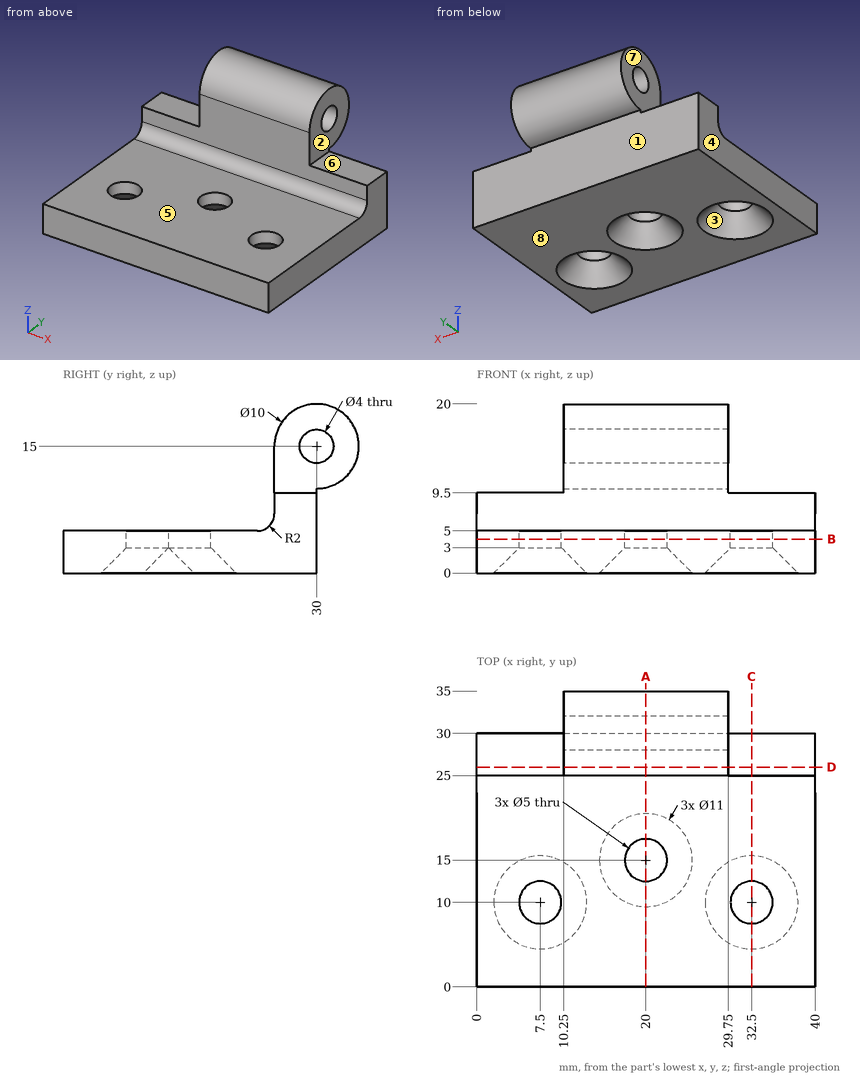
Study the drawing (mm; zero at the part's minimum x, y, z) and answer. A direction names the side the tool comes from. Round coordinates to 2 decimals unless told otherwise and drop trailing zeros. Loops run counter-clockwise (first coordinate to the right, second up) from the corner with the lowest first, then second, coordinate; pieces in that order, holes last.
Q1. Section C-C, the plane x = 32.5 is taken. Determine the outline of the cut face in (y, z), then the cut area to 3 significant figures.
Q2. Section D-D, the plane y = 26 is taken. Determine the outline of the cut face in (x, z), then the cut area to 3 significant figures.
Q3. Section B-B, the plane z = 4 is taken. Determine the outline of the cut face in (x, y), then the cut area to 3 significant figures.
Q4. Section A-A, the plane x = 20 is taken. Determine the outline of the cut face in (y, z).
Q5. For a pull along X with two mould halves and no side action, classify the marked faces 1, 2 and 3 as released by +X, released by -X, zero draft, split by the parting line, or undercut.
Q6. Given pin 1 Ø2.5 at (x, z) = (17, 11) entering from -Y; pin 2 Ø3 at (x, y) = (32.5, 10) entering from -Z; pin 3 Ø11 at (y, z) = (31, 15.5) entering from -X; pin 4 Ø4 at (x, y) = (4, 6.5) entering from +Z, each flat-ended and moving along its own axis, determine where each tip first touches the part or whether it passes through.
Q7. Which of the six approach directions +Z, -Z, +X, -X, +Y, -Y give full straight-line access (tool end or side, diameter ignored) to the marked faces 4, 5, 6, 7 and 8?
Q8. Find the intervals of material crossed by line 1 (X direction, y = 10, z = 3.4); line 2 (Y direction, x = 32.5, z = 4.55); line 3 (Y direction, x = 25.5, z = 15), in increasing order.
Completed:
1. outline: (0, 0) - (4.5, 0) - (7.5, 3) - (7.5, 5) - (0, 5) - close; (12.5, 3) - (15.5, 0) - (30, 0) - (30, 9.5) - (25, 9.5) - (25, 7) arc R2 cw to (23, 5) - (12.5, 5) - close
1. area: 139 mm2
2. outline: (0, 0) - (40, 0) - (40, 9.5) - (29.75, 9.5) - (29.75, 18) - (10.25, 18) - (10.25, 9.5) - (0, 9.5) - close
2. area: 546 mm2
3. outline: (0, 0) - (40, 0) - (40, 30) - (0, 30) - close; hole circle Ø5 at (7.5, 10); hole circle Ø5 at (20, 15); hole circle Ø5 at (32.5, 10)
3. area: 1,140 mm2
4. outline: (0, 0) - (9.5, 0) - (12.5, 3) - (12.5, 5) - (0, 5) - close; (17.5, 3) - (20.5, 0) - (30, 0) - (30, 10) arc R5 ccw (long way) to (25, 15) - (25, 7) arc R2 cw to (23, 5) - (17.5, 5) - close; hole circle Ø4 at (30, 15)
5. face 1: zero draft
5. face 2: released by +X
5. face 3: undercut
6. pin 1: stops at y = 25
6. pin 2: passes through
6. pin 3: stops at x = 10.25
6. pin 4: stops at z = 5
7. face 4: +Z, -Z, -X, +Y, -Y
7. face 5: +Z, +X, -X, -Y
7. face 6: +Z, +X, +Y, -Y
7. face 7: +Z, -X, +Y, -Y
7. face 8: -Z, +X, -X, +Y, -Y
8. line 1: x = 0 to 5, 10 to 30, 35 to 40
8. line 2: y = 0 to 7.5, 12.5 to 30
8. line 3: y = 25 to 28, 32 to 35
